Geometry: final body of the model. Coordinates: model frame, mm. Coordinates: 2 decimals unless noted, no trailing zeros. Order: outer loops, then holes, each group sorted by start corner. A loop starts at its lowest first (then second) coordinate and runs counter-clockwise, first axis right, second up. Notation, with made-up numbers: (83, 8) -> (142, 8) arc R19 cw to (142, 26) -> close; hole circle Ø8 at (66, -32). An arc over 180 degrees is marked (long way). Use one line per item in the form item = value.
```python
from build123d import *

# Parameters (mm, degrees)
BODYSKE_R    = 1.25
BODY_DEPTH   = 2
MODLUGSKE_R  = 1.25
MODLUG_DEPTH = 2


with BuildPart() as part:
    # BodySke → Body (new body)
    with BuildSketch(Plane.XY):
        with BuildLine():
            Line((6.15473831, -21.381807602), (4.998669473, -17.365578122))
            ThreePointArc((4.998669473, -17.365578122), (6.301661395, -14.225456519), (9.652536987, -14.799725088))
            ThreePointArc((9.652536987, -14.799725088), (11.602164826, -15.711310789), (13.605169738, -14.923904589))
            ThreePointArc((13.605169738, -14.923904589), (0, 18.15), (-13.605169738, -14.923904589))
            ThreePointArc((-13.605169738, -14.923904589), (-11.602164826, -15.711310789), (-9.652536987, -14.799725088))
            ThreePointArc((-9.652536987, -14.799725088), (-6.301661395, -14.225456519), (-4.998669473, -17.365578122))
            Line((-4.998669473, -17.365578122), (-6.15473831, -21.381807602))
            ThreePointArc((-6.15473831, -21.381807602), (0, 22.25), (6.15473831, -21.381807602))
        make_face()
        with Locations((7.617340292, -16.611795564)):
            Circle(BODYSKE_R, mode=Mode.SUBTRACT)
        with Locations((-7.617340292, -16.611795564)):
            Circle(BODYSKE_R, mode=Mode.SUBTRACT)
    extrude(amount=-BODY_DEPTH)

    # ModLugSke → ModLug (add, through all)
    with BuildSketch(Plane.XY):
        with BuildLine():
            Line((6.15473831, -21.381807602), (4.328974749, -15.039031805))
            ThreePointArc((4.328974749, -15.039031805), (4.337407237, -14.963258149), (4.396797536, -14.915450762))
            ThreePointArc((4.396797536, -14.915450762), (6.665405802, -14.049016531), (8.771452297, -12.839942547))
            ThreePointArc((8.771452297, -12.839942547), (8.837981797, -12.823028062), (8.899741793, -12.852994325))
            ThreePointArc((8.899741793, -12.852994325), (12.341754083, -14.219037165), (15.642102603, -12.539388009))
            Line((15.642102603, -12.539388009), (17.360405349, -13.916854031))
            ThreePointArc((17.360405349, -13.916854031), (12.335796621, -18.517306006), (6.15473831, -21.381807602))
        make_face()
        with Locations((7.617340292, -16.611795564)):
            Circle(MODLUGSKE_R, mode=Mode.SUBTRACT)
        with BuildLine():
            Line((-6.15473831, -21.381807602), (-4.328974749, -15.039031805))
            ThreePointArc((-4.328974749, -15.039031805), (-4.337407237, -14.963258149), (-4.396797536, -14.915450762))
            ThreePointArc((-4.396797536, -14.915450762), (-6.665405802, -14.049016531), (-8.771452297, -12.839942547))
            ThreePointArc((-8.771452297, -12.839942547), (-8.837981797, -12.823028062), (-8.899741793, -12.852994325))
            ThreePointArc((-8.899741793, -12.852994325), (-12.341754083, -14.219037165), (-15.642102603, -12.539388009))
            Line((-15.642102603, -12.539388009), (-17.360405349, -13.916854031))
            ThreePointArc((-17.360405349, -13.916854031), (-12.335796621, -18.517306006), (-6.15473831, -21.381807602))
        make_face()
        with Locations((-7.617340292, -16.611795564)):
            Circle(MODLUGSKE_R, mode=Mode.SUBTRACT)
    extrude(amount=-MODLUG_DEPTH)


solid = part.part
```
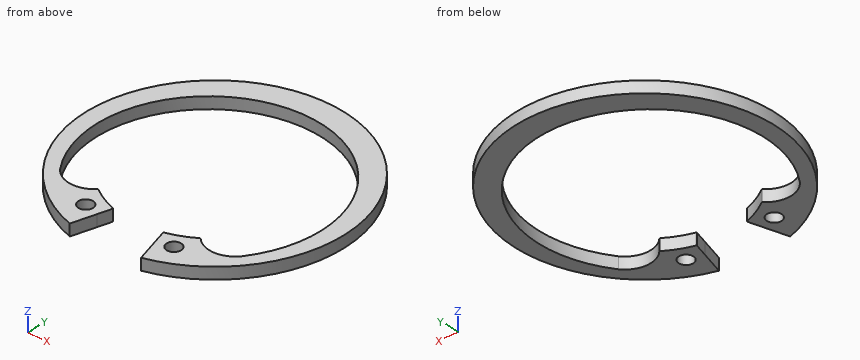
1) Section C-C, the plane y = -8. Output: boundary loops of the cut face in (x, z), and give its area (3 significant figures).
Results found:
outline = (-20.76, -2) -> (-18.09, -2) -> (-18.09, 0) -> (-20.76, 0) -> close; (18.09, -2) -> (20.76, -2) -> (20.76, 0) -> (18.09, 0) -> close
area = 10.7 mm2
2) Section A-A, the plane y = 4. Output: boundary loops of the cut face in (x, z).
Results found:
outline = (-21.89, -2) -> (-18.63, -2) -> (-18.63, 0) -> (-21.89, 0) -> close; (18.63, -2) -> (21.89, -2) -> (21.89, 0) -> (18.63, 0) -> close
3) Section B-B, the plane z = -1.3. Give the number of separate pieces and of enclosed holes in the cut face, and give its area (3 significant figures).
Results found:
separate_pieces = 1
enclosed_holes = 2
area = 421 mm2
4) Section D-D, the plane x = 0. Output: boundary loops of the cut face in (y, z), and give its area (3 significant figures).
Results found:
outline = (18.15, -2) -> (22.25, -2) -> (22.25, 0) -> (18.15, 0) -> close
area = 8.20 mm2
5) Material intervals for probe 1 along X at (y, z) = (-17, -1.3); probe 2 along X at (y, z) = (16, -1.7); probe 3 along X at (y, z) = (-12, -1.6), sorted ascending. Write a range as from..to.
Results found:
probe_1 = -14.35..-8.81, -6.43..-4.89, 4.89..6.43, 8.81..14.35
probe_2 = -15.46..-8.86, 8.86..15.46
probe_3 = -18.74..-16.03, 16.03..18.74
